Source: CAD feature listing. Evaluate the final solid. Frame: model axes, mm. Give positions to 0.01 mm unless a question says otherwise; leave off trailing zeros. Loops run counter-clockwise (first coordinate to the right, second up) from the corner with the lowest first, then second, coordinate; pieces in that order, holes last. Notation, with made-up numbers: (65.5, -14.5) -> (119.5, -14.5) arc R17 ccw to (119.5, 11.5) -> close; hole circle Ø2 at (78, 46). An arc over 180 degrees is marked (long way). Put each result on its own line as item: value.
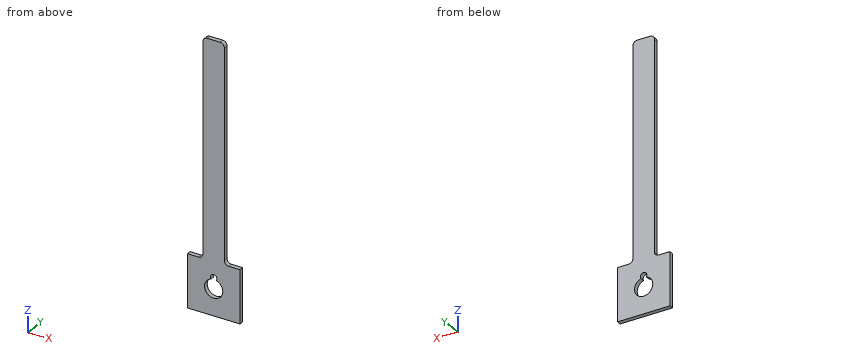
Autodesk Inventor part; units mm, degrees
ref_plane "YZ Plane" through (0, 0, 0) normal (1, 0, 0) x (0, 1, 0)
ref_plane "XZ Plane" through (0, 0, 0) normal (0, 1, 0) x (-1, 0, 0)
ref_plane "XY Plane" through (0, 0, 0) normal (0, 0, 1) x (1, 0, 0)
sketch "Sketch1" plane through (0, 0, 0) normal (0, 1, 0) x (-1, 0, 0)
  circle A0 centre (0, 0) radius 4.25
  line L0 (-12.25, -12.25) -> (12.25, -12.25)
  line L1 (12.25, -12.25) -> (12.25, 12.25)
  line L2 (12.25, 12.25) -> (-12.25, 12.25)
  line L3 (-12.25, 12.25) -> (-12.25, -12.25)
  line L4 (-12.25, -12.25) -> (12.25, 12.25) construction
  line L5 (12.25, -12.25) -> (-12.25, 12.25) construction
  dimension "d0" = 24.5
  dimension "d1" = 8.5
extrude "Extrusion1" add sketch "Sketch1" along normal blind 2
sketch "Sketch2" plane through (0, 2, 0) normal (0, 1, 0) x (1, 0, 0)
  circle A0 centre (0, -4.9582) radius 1.5
  point P0 (0, 0)
  dimension "d4" = 3
extrude "Extrusion2" cut sketch "Sketch2" against normal blind 3
sketch "Sketch3" plane through (0, 2, 0) normal (0, 1, 0) x (1, 0, 0)
  line L0 (-12.25, -12.25) -> (12.25, -12.25)
  line L1 (5, -112.25) -> (-5, -112.25)
  line L2 (-5, -112.25) -> (-5, -12.25)
  line L3 (-5, -12.25) -> (5, -12.25)
  line L4 (5, -12.25) -> (5, -112.25)
  line L5 (5, -112.25) -> (-5, -12.25) construction
  line L6 (-5, -112.25) -> (5, -12.25) construction
  point P0 (0, 0)
  point P1 (0, -62.25)
  point P2 (0, -62.25)
  point P3 (5, -12.25)
  dimension "d7" = 100
  dimension "d8" = 10
extrude "Extrusion3" add sketch "Sketch3" against normal up to surface (2 mm away)
fillet "Fillet1" radius 2 4 edges at (5, 1, 12.25) (-5, 1, 12.25) (5, 1, 112.25) (-5, 1, 112.25)
equation "\"d5\" = d4"
properties part number "pb_hole_stick" material "Lead"
(1) Section C-C on y = 1.6. Return loops of the section in (x, z), then the cut area to 3 significant figures.
Calculated:
outline: (-12.25, -12.25) -> (12.25, -12.25) -> (12.25, 12.25) -> (7, 12.25) arc R2 cw to (5, 14.25) -> (5, 110.25) arc R2 ccw to (3, 112.25) -> (-3, 112.25) arc R2 ccw to (-5, 110.25) -> (-5, 14.25) arc R2 cw to (-7, 12.25) -> (-12.25, 12.25) -> close; hole (-1.21, 4.07) arc R4.25 ccw (long way) to (1.21, 4.07) arc R1.5 ccw (long way) to start
area: 1,540 mm²
(2) Line query: probe 1 along Z at (x, y) = (0, 0.65); probe 2 along X at (y, z) = (0.85, 0); probe 3 along X at (y, z) = (1.2, 105.5). Output: solid intervals per line, ascending. Write a range as from..to.
Calculated:
probe 1: z = -12.25..-4.25, 6.46..112.25
probe 2: x = -12.25..-4.25, 4.25..12.25
probe 3: x = -5..5
(3) Section D-D on x = 10. Return loops of the section in (y, z).
Calculated:
outline: (0, -12.25) -> (2, -12.25) -> (2, 12.25) -> (0, 12.25) -> close
(4) Section A-A on z = 0. Return loops of the section in (x, y).
Calculated:
outline: (-12.25, 0) -> (-4.25, 0) -> (-4.25, 2) -> (-12.25, 2) -> close; (4.25, 0) -> (12.25, 0) -> (12.25, 2) -> (4.25, 2) -> close
(5) First-contact query: P1, Ø1, axis at y = 1, z = 78, coming from the +X side; P2, Ø5, axis at x = -1.5, z = 68.5, coming from the -Y side; P3, Ø0.6, axis at x = -8.5, y = 0.5, coming from the +Z side. Flat tips, straight axial feed; report the tip coordinate or a pass-through.
Calculated:
P1: stops at x = 5
P2: stops at y = 0
P3: stops at z = 12.25
(6) Section B-B on x = 0. Return loops of the section in (y, z), then the cut area to 3 significant figures.
Calculated:
outline: (0, -12.25) -> (2, -12.25) -> (2, -4.25) -> (0, -4.25) -> close; (0, 6.46) -> (2, 6.46) -> (2, 112.25) -> (0, 112.25) -> close
area: 228 mm²
